```python
from build123d import *

# Parameters (mm, degrees)
BOSS_EXTRUDE1_DEPTH   = 20
BOSS_EXTRUDE1_2_DEPTH = 20
BOSS_EXTRUDE1_3_DEPTH = 20
BOSS_EXTRUDE1_4_DEPTH = 20
BOSS_EXTRUDE2_DEPTH   = 12
SKETCH5_W             = 25
SKETCH5_H             = 40
SKETCH5_W_2           = 40
SKETCH5_H_2           = 25
CUT_EXTRUDE1_DEPTH    = 5


with BuildPart() as part:
    # Sketch2 → Boss-Extrude1 (new body)
    with BuildSketch(Plane.XY):
        Polygon((110, 10), (123.5, 10), (123.5, -10), (110, -10), (110, -5.5), (114.5, -5.5), (121, -5.5), (121, 5.5), (114.5, 5.5), (110, 5.5), align=None)
    extrude(amount=BOSS_EXTRUDE1_DEPTH)



with BuildPart() as body_2:
    # Sketch2 → Boss-Extrude1 2 (new body)
    with BuildSketch(Plane.XY):
        Polygon((10, -110), (10, -123.5), (-10, -123.5), (-10, -110), (-5.5, -110), (-5.5, -114.5), (-5.5, -121), (5.5, -121), (5.5, -114.5), (5.5, -110), align=None)
    extrude(amount=BOSS_EXTRUDE1_2_DEPTH)


with BuildPart() as body_3:
    # Sketch2 → Boss-Extrude1 3 (new body)
    with BuildSketch(Plane.XY):
        Polygon((-110, -10), (-123.5, -10), (-123.5, 10), (-110, 10), (-110, 5.5), (-114.5, 5.5), (-121, 5.5), (-121, -5.5), (-114.5, -5.5), (-110, -5.5), align=None)
    extrude(amount=BOSS_EXTRUDE1_3_DEPTH)


with BuildPart() as body_4:
    # Sketch2 → Boss-Extrude1 4 (new body)
    with BuildSketch(Plane.XY):
        Polygon((-10, 110), (-5.5, 110), (-5.5, 114.5), (-5.5, 121), (5.5, 121), (5.5, 114.5), (5.5, 110), (10, 110), (10, 123.5), (-10, 123.5), align=None)
    extrude(amount=BOSS_EXTRUDE1_4_DEPTH)


with BuildPart() as part_1:
    add(part.part)

    add(body_2.part)  # Boss-Extrude2 merges body 2

    add(body_3.part)  # Boss-Extrude2 merges body 3

    add(body_4.part)  # Boss-Extrude2 merges body 4
    # Sketch3 → Boss-Extrude2 (add)
    with BuildSketch(Plane(origin=(0, 0, 0), x_dir=(-1, 0, 0), z_dir=(0, 0, -1))):
        with BuildLine():
            Line((10, 123.5), (-10, 123.5))
            ThreePointArc((-10, 123.5), (-87.613497819, 87.613497819), (-123.5, 10))
            Line((-123.5, 10), (-123.5, -10))
            ThreePointArc((-123.5, -10), (-87.613497819, -87.613497819), (-10, -123.5))
            Line((-10, -123.5), (10, -123.5))
            ThreePointArc((10, -123.5), (87.613497819, -87.613497819), (123.5, -10))
            Line((123.5, -10), (123.5, 10))
            ThreePointArc((123.5, 10), (87.613497819, 87.613497819), (10, 123.5))
        make_face()
        with BuildLine():
            ThreePointArc((-110, 10), (-103.205416168, 39.352789909), (-88.731734836, 65.777497923))
            Line((-88.731734836, 65.777497923), (-80.698341025, 59.822283075))
            ThreePointArc((-80.698341025, 59.822283075), (-72.199580711, 69.843742323), (-62.465465553, 78.670155776))
            Line((-62.465465553, 78.670155776), (-68.683805088, 86.501646913))
            ThreePointArc((-68.683805088, 86.501646913), (-41.058841255, 102.538634449), (-10, 110))
            Line((-10, 110), (10, 110))
            ThreePointArc((10, 110), (39.352789909, 103.205416168), (65.777497923, 88.731734836))
            Line((65.777497923, 88.731734836), (59.822283075, 80.698341025))
            ThreePointArc((59.822283075, 80.698341025), (69.843742323, 72.199580711), (78.670155776, 62.465465553))
            Line((78.670155776, 62.465465553), (86.501646913, 68.683805088))
            ThreePointArc((86.501646913, 68.683805088), (102.538634449, 41.058841255), (110, 10))
            Line((110, 10), (110, -10))
            ThreePointArc((110, -10), (103.205416168, -39.352789909), (88.731734836, -65.777497923))
            Line((88.731734836, -65.777497923), (80.698341025, -59.822283075))
            ThreePointArc((80.698341025, -59.822283075), (72.199580711, -69.843742323), (62.465465553, -78.670155776))
            Line((62.465465553, -78.670155776), (68.683805088, -86.501646913))
            ThreePointArc((68.683805088, -86.501646913), (41.058841255, -102.538634449), (10, -110))
            Line((10, -110), (-10, -110))
            ThreePointArc((-10, -110), (-39.352789909, -103.205416168), (-65.777497923, -88.731734836))
            Line((-65.777497923, -88.731734836), (-59.822283075, -80.698341025))
            ThreePointArc((-59.822283075, -80.698341025), (-69.843742323, -72.199580711), (-78.670155776, -62.465465553))
            Line((-78.670155776, -62.465465553), (-86.501646913, -68.683805088))
            ThreePointArc((-86.501646913, -68.683805088), (-102.538634449, -41.058841255), (-110, -10))
            Line((-110, -10), (-110, -5.5))
            Line((-110, -5.5), (-110, 5.5))
            Line((-110, 5.5), (-110, 10))
        make_face(mode=Mode.SUBTRACT)
    extrude(amount=BOSS_EXTRUDE2_DEPTH)

    # Sketch5 → Cut-Extrude1 (cut)
    with BuildSketch(Plane(origin=(0, 0, -12), x_dir=(-1, 0, 0), z_dir=(0, 0, -1))):
        with Locations((-116.75, 0)):
            Rectangle(SKETCH5_W, SKETCH5_H)
        with Locations((0, 116.75)):
            Rectangle(SKETCH5_W_2, SKETCH5_H_2)
        with Locations((116.75, 0)):
            Rectangle(SKETCH5_W, SKETCH5_H)
        with Locations((0, -116.75)):
            Rectangle(SKETCH5_W_2, SKETCH5_H_2)
    extrude(amount=-CUT_EXTRUDE1_DEPTH, mode=Mode.SUBTRACT)


solid = part_1.part
```
Design review of the part built by this model. Coordinates are the model's own, in mm. A direction names the side the tool comes from. Give positions to 0.01 mm unless a question says otherwise; leave off trailing zeros. Order: outer loops, then holes, each group sorted by start corner. A loop starts at its lowest first (then second) coordinate and runs counter-clockwise, first axis right, second up. Notation, with made-up numbers: (72, -15.5) -> (86, -15.5) arc R18 ccw to (86, 7.5) -> close; hole circle Ø11 at (-29.5, 34.25). An arc over 180 degrees is marked (long way). Write each question's results on one line, items separated by ' | '. Start each with the question number.
Q1. Wall thickness on L1, parallel to Z at x = 86, y = 87; L2, parallel to Y at x = 42.5, z = -1.5; L3, parallel to Y at x = 13, z = -5: over which ranges is each line inside the solid? List them lowest first. Write a range as from..to.
Q2. Machinability: for faces 4 (the flat face through (117, 10, 10)), 5 (the flat face through (0, -116, -7)), 6 (the flat face through (-75, -75, 0)), 7 (the flat face through (-82.53, 65.53, -5.92)), 8 (the flat face through (-115, 0, 0)), which of the approach directions +Z, -Z, +X, -X, +Y, -Y give a long, thin tool a straight path to every point of the face, cutting with its end or side? Answer none if there is none.
Q3. For pin 1 (7 mm diameter, centred on x = 120, z = 5, fed in from -Y); pin 2 (16.5 mm diameter, centred on x = -118, y = 2, fed in from -Z); pin 3 (3.5 mm diameter, centred on y = 114, z = 12.5, fed in from -X), all flat-tipped, find the tip position at first contact; note any pin that passes through.
Q4. Mouldability with a two-part tool opening along X and no side actions: class faces 1 (the flat face through (0.1, -121.2, 20)), 2 (the flat face through (-10, -117, 10)), 3 (the flat face through (-121, 0, 10)) as +X half, -X half, draft (parallel to the pull), parting line (faces both ways), or undercut.
Q5. Add section C-C on x = -34. Give the boundary of the cut face in (y, z), and give its area (3 significant figures).
Q6. Add section A-A on z = 10.5. State how many separate pieces and enclosed holes the cut face has, and give its area (3 significant figures).
Q7. Add section B-B on y = -41.5. Give the boundary of the cut face in (x, z), and give its area (3 significant figures).
Found:
1) L1: z = -12..0 | L2: y = -116.39..-101.95, 101.95..116.39 | L3: y = -123.22..-109.69, 109.69..123.22
2) face 4: +Z, +X, -X, +Y | face 5: -Z, +Y, -Y | face 6: +Z, -X, -Y | face 7: +Z, -Z | face 8: +Z
3) pin 1: stops at y = -10 | pin 2: stops at z = -7 | pin 3: stops at x = -10
4) face 1: draft | face 2: -X half | face 3: undercut
5) outline: (-119.15, -12) -> (-105.09, -12) -> (-105.09, 0) -> (-119.15, 0) -> close; (105.09, -12) -> (119.15, -12) -> (119.15, 0) -> (105.09, 0) -> close | area: 337 mm2
6) separate pieces: 4 | enclosed holes: 0 | area: 596 mm2
7) outline: (-116.75, -12) -> (-102.36, -12) -> (-102.36, 0) -> (-116.75, 0) -> close; (102.36, -12) -> (116.75, -12) -> (116.75, 0) -> (102.36, 0) -> close | area: 345 mm2
